```python
from build123d import *

# Parameters (mm, degrees)
BOSS_EXTRUDE1_DEPTH = 3.048
CUT_EXTRUDE1_REACH  = 5.048
SKETCH2_R           = 2.921


with BuildPart() as part:
    # Sketch1 → Boss-Extrude1 (new body)
    with BuildSketch(Plane.XY):
        Polygon((130.175, 0), (130.175, 5.9944), (168.275, 5.9944), (168.275, 0), (298.45, 0), (298.45, 63.5), (295.402, 63.5), (295.402, 126.929256228), (298.45, 126.929256228), (298.45, 190.429256228), (295.402, 190.429256228), (295.402, 253.929256228), (236.3216, 253.929256228), (236.3216, 247.960256228), (177.2412, 247.960256228), (177.2412, 253.929256228), (118.1608, 253.929256228), (118.1608, 247.960256228), (59.0804, 247.960256228), (59.0804, 253.929256228), (-5.9944, 253.929256228), (-5.9944, 190.5), (0, 190.5), (0, 127), (-5.9944, 127), (-5.9944, 63.5), (0, 63.5), (0, 0), align=None)
    extrude(amount=BOSS_EXTRUDE1_DEPTH)

    # Sketch2 → Cut-Extrude1 (cut, up to next)
    with BuildSketch(Plane.XY.offset(3.048), mode=Mode.PRIVATE) as cut_extrude1_sk1:
        with Locations((12.7, 38.1)):
            Circle(SKETCH2_R)
    cut_extrude1_tool1 = extrude(cut_extrude1_sk1.sketch, amount=-CUT_EXTRUDE1_REACH, mode=Mode.PRIVATE) & part.part
    add(cut_extrude1_tool1.solids().sort_by_distance((12.7, 38.1, 3.048))[0], mode=Mode.SUBTRACT)


solid = part.part
```
Can you work these out from the model? Positions are in its coordinate system, mm. Round coordinates to 2 decimals unless told otherwise and drop trailing zeros. Loops run counter-clockwise (first coordinate to the right, second up) from the corner with the lowest first, then second, coordinate; pieces in that order, holes last. Notation, with made-up numbers: M -32,79 L -6,79 A16 cw -6,109 Z; hole C 84.25,33.25 d3. An arc over 180 degrees is marked long. Write item = value, one per line. Start each with the question number.
(1) I need wall thicknesses on line 1 along Y through (x, z) = (12.7, 1.8); line 2 along X through (y, z) = (76, 2.2); line 3 along X through (y, z) = (42, 0.8). Which ranges of each line are inside material? Lowest first, please.
(2) Suppose I cut it at C-C on y = 152. Write out the boundary of the cut face in (x, z), plus the area to 3 significant figures.
(3) Suppose I cut it at B-B on x = 135. Write out the boundary of the cut face in (y, z).
(4) I'm going to push flat-ended pins straight in: P1, Ø0.9, axis at y = 17.5, z = 2, coming from the -X side; P2, Ø1.5, axis at x = -4, z = 1.5, coming from the -Y side; P3, Ø1.5, axis at y = 251, z = 1, coming from the +X side. Where does each tip first touch, or does it pass through?
Answer block:
q1.line_1 = 0 to 35.18, 41.02 to 253.93
q1.line_2 = -5.99 to 295.4
q1.line_3 = 0 to 298.45
q2.outline = M 0,0 L 298.45,0 L 298.45,3.05 L 0,3.05 Z
q2.area = 910 mm²
q3.outline = M 5.99,0 L 253.93,0 L 253.93,3.05 L 5.99,3.05 Z
q4.P1 = 0
q4.P2 = 63.5
q4.P3 = 295.4
